Build history of the part. All positions in model axes, mm. Face numbers are marked on the shaded views. A direction names the side the tool comes from. Give positions to 0.01 mm unless a question says otherwise; leave off trailing zeros. Order: outer loops, then holes, each group sorted by start corner. A loop starts at its lowest first (then second) coordinate and runs counter-clockwise, first axis right, second up. Notation, with made-up numbers: M -15,-30.75 L 36,-30.75 A15 cw 36,-21.75 Z; hole C -35,23.25 d1. An arc over 180 degrees is marked long. One line per item, written item: value. Start each with the question number.
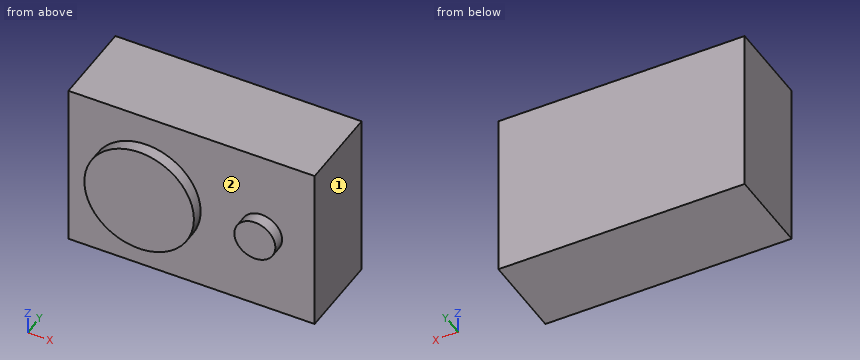
from build123d import *

# Parameters (mm, degrees)
F0_W     = 60
F0_H     = 41
F1_DEPTH = 21
F2_R     = 13.3531025353
F2_R_2   = 5
F3_DEPTH = 3


# Not quite as in the source:
# - a feature names something its author has since deleted; it is built from what else it names


with BuildPart() as f1:
    # F0 (on Front) → F1 (new body)
    with BuildSketch(Plane.XZ):
        Rectangle(F0_W, F0_H)
    extrude(amount=F1_DEPTH)

    # F2 (on face) → F3 (join)
    with BuildSketch(Plane.XZ.offset(21)):
        with Locations((-11.1307431944, -0.2782683878)):
            Circle(F2_R)
        with Locations((17.0671385713, -0.2782683878)):
            Circle(F2_R_2)
    extrude(amount=F3_DEPTH)


solid = f1.part
1) Slice it at B-B (z = -1). List the corners of the cut face in (x, y), plus the area to 3 significant figures.
2) Slice it at C-C (x = -23.5). List the corners of the cut face in (y, z).
3) Slice it at D-D (x = 23). List the corners of the cut face in (y, z).
4) Drop a flat-ended pin along its axis: P1, Ø2, axis at x = 6.5, z = 3.5, coming from the -Y side. Give the stop position or say it passes through.
5) Slice it at A-A (x = 17). List the corners of the cut face in (y, z).
6) Tool access for the marked faces 1 and 2: list every direction of +Z, -Z, +X, -X, +Y, -Y with a clear straight run to the whole face (end or side of a thin tool).
7) Drill centre lines: line 1 (Y direction, x = 4, z = 14); line 2 (Z direction, x = -3.5, y = -22.75). Where is each one in solid material? Low to high.
Results list:
1. outline: M -30,-21 L -24.46,-21 L -24.46,-24 L 2.2,-24 L 2.2,-21 L 12.12,-21 L 12.12,-24 L 22.01,-24 L 22.01,-21 L 30,-21 L 30,0 L -30,0 Z
1. area: 1,370 mm²
2. outline: M -24,-5.31 L -21,-5.31 L -21,-20.5 L 0,-20.5 L 0,20.5 L -21,20.5 L -21,4.75 L -24,4.75 Z
3. outline: M -21,-20.5 L 0,-20.5 L 0,20.5 L -21,20.5 Z
4. P1: stops at y = -21
5. outline: M -24,-5.28 L -21,-5.28 L -21,-20.5 L 0,-20.5 L 0,20.5 L -21,20.5 L -21,4.72 L -24,4.72 Z
6. face 1: +Z, -Z, +X, +Y, -Y
6. face 2: -Y
7. line 1: y = -21 to 0
7. line 2: z = -11.24 to 10.68
